Verification items for the finished model (mm, model axes). A direction names the side the tool comes from. Give positions to 0.01 mm unless a question says otherwise; leave off trailing zeros. Write each loop counter-clockwise with the first axis right and the second up, starting at its lowest first coordinate (ties: lowest second). Pieces come first, ordered by that corner, then holes. Notation, with made-up numbers: (-40, 63) - (2, 63) arc R33 cw to (2, 102) - close; hole circle Ø10 at (-17, 77). An arc over 180 degrees is marked (long way). Put each result on its own line as item: value.
from build123d import *

# Parameters (mm, degrees)
BOSS_EXTRUDE1_DEPTH = 10
CUT_EXTRUDE2_DEPTH  = 11
SKETCH3_W           = 0.65
SKETCH3_H           = 4
CUT_EXTRUDE3_DEPTH  = 7.45


with BuildPart() as part:
    # Sketch1 → Boss-Extrude1 (new body)
    with BuildSketch(Plane(origin=(0, 0, 0), x_dir=(1, 0, 0), z_dir=(0, 1, 0))):
        Polygon((1.5, 1.75), (3.5, 1.75), (3.5, 0), (-3.5, 0), (-3.5, 1.75), (-1.5, 1.75), (-1.5, 6.75), (1.5, 6.75), (23.5, 6.75), (26.5, 6.75), (26.5, 1.75), (28.5, 1.75), (28.5, 0), (21.5, 0), (21.5, 1.75), (23.5, 1.75), (23.5, 4.75), (1.5, 4.75), align=None)
    extrude(amount=BOSS_EXTRUDE1_DEPTH)

    # Sketch2 → Cut-Extrude2 (cut, through all)
    with BuildSketch(Plane(origin=(0, 10, 0), x_dir=(1, 0, 0), z_dir=(0, 1, 0))):
        Polygon((-3.65, 1.9), (-3.65, -0.15), (3.65, -0.15), (3.65, 1.9), (1.65, 1.9), (1.65, 4.6), (23.35, 4.6), (23.35, 1.9), (21.35, 1.9), (21.35, -0.15), (28.65, -0.15), (28.65, 1.9), (26.65, 1.9), (26.65, 6.9), (-1.65, 6.9), (-1.65, 1.9), align=None)
        Polygon((-3.35, 1.6), (-3.35, 0.15), (3.35, 0.15), (3.35, 1.6), (1.35, 1.6), (1.35, 4.9), (23.65, 4.9), (23.65, 1.6), (21.65, 1.6), (21.65, 0.15), (28.35, 0.15), (28.35, 1.6), (26.35, 1.6), (26.35, 6.6), (-1.35, 6.6), (-1.35, 1.6), align=None, mode=Mode.SUBTRACT)
    extrude(amount=-CUT_EXTRUDE2_DEPTH, mode=Mode.SUBTRACT)

    # Sketch3 → Cut-Extrude3 (cut, through all)
    with BuildSketch(Plane(origin=(0, 0, -6.6), x_dir=(-1, 0, 0), z_dir=(0, 0, -1))):
        with Locations((-12.5, 5)):
            Rectangle(SKETCH3_W, SKETCH3_H)
    extrude(amount=-CUT_EXTRUDE3_DEPTH, mode=Mode.SUBTRACT)


solid = part.part
Q1. Scan lines: line 1 along Z through (x, y) = (23, 5); line 2 along X through (y, z) = (0.5, -2.25); line 3 along Z through (x, y) = (19, 3). Record each from-to range of solid material in increasing order.
Answers follow:
line 1: z = -6.6 to -4.9, -1.6 to -0.15
line 2: x = -1.35 to 1.35, 23.65 to 26.35
line 3: z = -6.6 to -4.9
Q2. Section check A-A, the plane y = 5.75. Record the cut outline in (x, z) (3 decimals), plus the area to 3 significant figures.
Answers follow:
outline: (-3.35, -1.6) - (-1.35, -1.6) - (-1.35, -6.6) - (12.175, -6.6) - (12.175, -4.9) - (1.35, -4.9) - (1.35, -1.6) - (3.35, -1.6) - (3.35, -0.15) - (-3.35, -0.15) - close; (12.825, -6.6) - (26.35, -6.6) - (26.35, -1.6) - (28.35, -1.6) - (28.35, -0.15) - (21.65, -0.15) - (21.65, -1.6) - (23.65, -1.6) - (23.65, -4.9) - (12.825, -4.9) - close
area: 83.2 mm2
Q3. Section check D-D, the plane z = -5.25. Record the cut outline in (x, y) (3 decimals), plus the area to 3 significant figures.
Answers follow:
outline: (-1.35, 0) - (26.35, 0) - (26.35, 10) - (-1.35, 10) - close; hole (12.175, 3) - (12.825, 3) - (12.825, 7) - (12.175, 7) - close
area: 274 mm2
Q4. Set-up check for faces 1 (the face through (-1.35, 5, -4)), 2 (the face through (27, 5, -1.6)), 3 (the face through (3.35, 5, -1)): record each of +Z, -Z, +X, -X, +Y, -Y from which the full face is reachable in a straight line by a thin tool's end or side.
Answers follow:
face 1: -Z, -X, +Y, -Y
face 2: -Z, +X, +Y, -Y
face 3: +Z, +Y, -Y
Q5. Release check for a two-part mould opening along X. For faces 4 (the face through (26.35, 5, -4)), 5 (the face through (12.175, 5, -6)), 6 (the face through (-2, 5, -1.6)) record: released by +X, released by -X, zero draft, split by the parting line, or undercut.
Answers follow:
face 4: released by +X
face 5: undercut
face 6: zero draft
Q6. Go/stop test with flat-tipped pins: pin 1 Ø1.4 at (y, z) = (5.5, -5.5) entering from +X; pin 2 Ø1.4 at (y, z) = (6, -5.5) entering from -X. Record where each tip stops, or that it passes through.
Answers follow:
pin 1: stops at x = 26.35
pin 2: stops at x = -1.35
Q7. Section check C-C, the plane z = -0.5. Record the cut outline in (x, y).
Answers follow:
outline: (-3.35, 0) - (3.35, 0) - (3.35, 10) - (-3.35, 10) - close; (21.65, 0) - (28.35, 0) - (28.35, 10) - (21.65, 10) - close
Q8. Section check B-B, the plane x = 3. Record the cut outline in (y, z).
Answers follow:
outline: (0, -6.6) - (10, -6.6) - (10, -4.9) - (0, -4.9) - close; (0, -1.6) - (10, -1.6) - (10, -0.15) - (0, -0.15) - close
